For this review, take the finished solid that the model builds, in its own axes (mm). Face numbers are marked on the shaded views. A direction names the side the tool comes from. Coordinates: 2 decimals unless noted, no trailing zeros. Write each question's results on one line, items separated by ' | '. Start each with the question number.
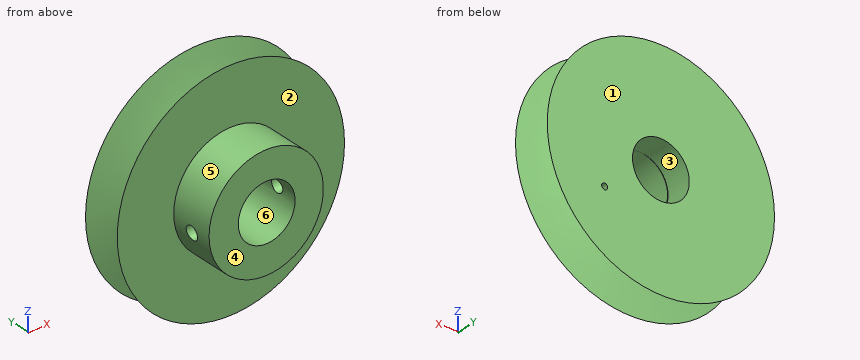
```python
from build123d import *

# Parameters (mm, degrees)
SKETCH117_R           = 3.25
CUT_EXTRUDE4_DEPTH    = 3
SKETCH122_R           = 6.539767279
BOSS_EXTRUDE1_DEPTH   = 5
M2X0_4_TAPPED_HOLE1_D = 1.6
SKETCH125_R           = 3.25
CUT_EXTRUDE5_DEPTH    = 7
SKETCH126_R           = 0.35
CUT_EXTRUDE6_DEPTH    = 2


with BuildPart() as part:
    # Sketch9 → Revolve1 (revolve)
    with BuildSketch(Plane.XY):
        with BuildLine():
            Line((-4.703089141, -2.935363462), (8.296910859, -2.935363462))
            Line((8.296910859, -2.935363462), (8.296910859, 1.564636538))
            Line((8.296910859, 1.564636538), (-4.703089141, 1.564636538))
            add(Edge.make_bspline(
                [(-4.703089141, 1.564636538), (8.296910859, -1.435363462), (-4.703089141, -2.935363462)],
                knots=[0, 0, 0, 1, 1, 1], degree=2))
        make_face()
    revolve(axis=Axis((8.296910859, -2.935363462, 0), (0, 1, 0)))

    # Sketch117 → Cut-Extrude4 (cut)
    with BuildSketch(Plane(origin=(0, 1.564636538, 0), x_dir=(1, 0, 0), z_dir=(0, 1, 0))):
        with Locations((8.29691086, 0)):
            Circle(SKETCH117_R)
    extrude(amount=-CUT_EXTRUDE4_DEPTH, mode=Mode.SUBTRACT)

    # Sketch122 → Boss-Extrude1 (add)
    with BuildSketch(Plane(origin=(0, -2.935363462, 0), x_dir=(-1, 0, 0), z_dir=(0, -1, 0))):
        with Locations((-8.29691086, 0)):
            Circle(SKETCH122_R)
    extrude(amount=BOSS_EXTRUDE1_DEPTH)

    # M2x0.4 Tapped Hole1 (through all)
    with Locations(Plane(origin=(1.815385484, -5.431649491, -0.870852953), x_dir=(0.133162682, 0, -0.991094193), z_dir=(-0.991094193, 0, -0.133162682))):
        with Locations((0, 0)):
            Hole(M2X0_4_TAPPED_HOLE1_D / 2)

    # Sketch125 → Cut-Extrude5 (cut)
    with BuildSketch(Plane(origin=(0, -1.435363462, 0), x_dir=(1, 0, 0), z_dir=(0, 1, 0))):
        with Locations((8.350281981, 0)):
            Circle(SKETCH125_R)
    extrude(amount=-CUT_EXTRUDE5_DEPTH, mode=Mode.SUBTRACT)

    # Sketch126 → Cut-Extrude6 (cut)
    with BuildSketch(Plane(origin=(0, 1.564636538, 0), x_dir=(1, 0, 0), z_dir=(0, 1, 0))):
        with Locations((14.730684235, 4.136659271)):
            Circle(SKETCH126_R)
    extrude(amount=-CUT_EXTRUDE6_DEPTH, mode=Mode.SUBTRACT)


solid = part.part
```
Q1. The part is to be moulded in two halves that separate along X. For the marked faces 4, 5 and 6, say which applies: pulls with the +X half, pulls with the -X half, needs draft (parallel to the pull), parting line crosses it, or undercut.
Q2. For the marked faces 1, 2 and 3, list the 3-axis set-ups (+Z, -Z, +X, -X, +Y, -Y) from which the entire face can be reached by the end or side of a thin tool; tool diameter is ignored.
Q3. Take a section at A-A, the plane z = -1. Give the number of separate pieces and of enclosed holes in the cut face, then the cut area to 3 significant figures.
Q4. To check wall thickness, follow line 1 along X through (y, z) = (-4, 0); line 2 along Z through (x, y) = (8.5, -4.75); line 3 along Y through (x, z) = (17.75, -3). State the ranges of each line that lie inside material, in increasing order.
Results:
1) face 4: needs draft | face 5: parting line crosses it | face 6: undercut
2) face 1: +Z, -Z, +X, -X, +Y | face 2: -Y | face 3: +Y
3) separate pieces: 3 | enclosed holes: 0 | area: 78.5 mm^2
4) line 1: 1.76 to 5.1, 11.6 to 14.84 | line 2: -6.54 to -3.25, 3.25 to 6.54 | line 3: -2.94 to -2.49, 0.77 to 1.56
